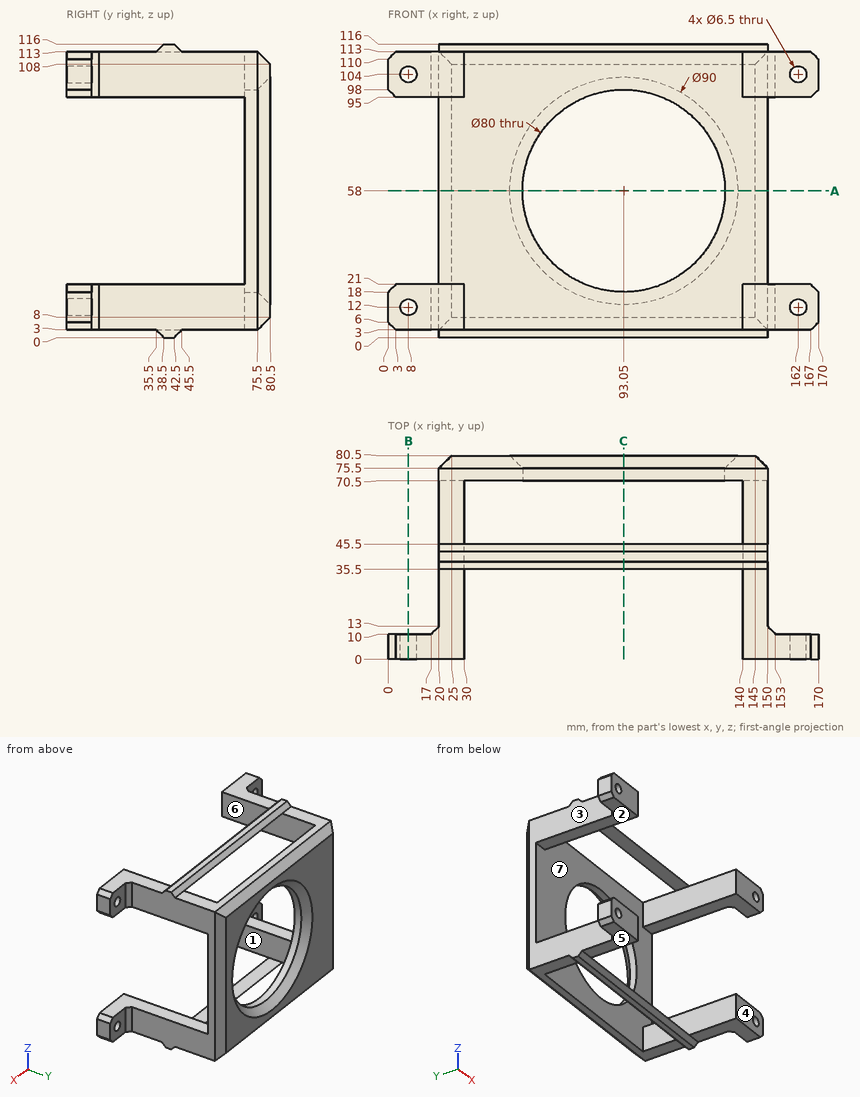
Study the drawing (mm; zero at the part's minimum x, y, z) and answer. A direction names the side the tool comes from. Round coordinates to 2 decimals unless told otherwise and drop trailing zeros. Write each loop counter-clockwise with the first axis right and the second up, starting at its lowest first coordinate (ties: lowest second). Pieces come first, ordered by that corner, then holes. Notation, with made-up numbers: (-34, -23.75) -> (-11, -23.75) arc R17 ccw to (-11, -12.75) -> close; hole circle Ø9 at (41.5, 30). An arc over 180 degrees is marked (long way). Answer as CSV lines item,"result". Start each with the question number.
(1) A tool of negligible diameter and unlimited length cuts with its end or side. For the marked faces 1, 2 and 3, from which of +Z, -Z, +X, -X, +Y, -Y can it reach the whole face along a straight path? Write none if from no direction.
(2) Each of these flat-tipped pins is pushed along its axis until it touches: pin 1 (18.5 mm diameter, centred on x = 9, z = 8.5, fed in from +Y); pin 2 (9 mm diameter, centred on y = 49, z = 101.5, fed in from +X); pin 3 (24 mm diameter, centred on x = 71, y = 67, fed in from +Z). Where does it stop, or does it pass through?
(3) The part is cut by section B-B, the plane x = 8. Give the vertices of the cut face in (y, z).
(4) The part is cut by section C-C, the plane x = 93.05. Give the number of separate pieces and of enclosed holes in the cut face, then the cut area to 3 significant figures.
(5) The part is cut by section A-A, the plane z = 58. Give the vertices of the cut face in (x, y), then the cut area to 3 significant figures.
(6) The mould has two halves that part along Z. Classify the marked faces 4, 5, 6 and 7: +Z half, -Z half, draft (parallel to the pull), parting line (faces both ways), or undercut.
(7) Find the intervals of material crossed by probe 1 along Z at (x, y) = (93.05, 73.5); probe 2 along X at (y, z) = (68.5, 14); probe 3 along Z at (x, y) = (25, 26.5), in increasing order.
Output values:
1,face 1,"-Y"
1,face 2,"+X, -X, -Y"
1,face 3,"+Z, -Z, -X, +Y"
2,pin 1,"stops at y = 11.25"
2,pin 2,"stops at x = 150"
2,pin 3,"stops at z = 113"
3,outline,"(0, 3) -> (10, 3) -> (10, 8.75) -> (0, 8.75) -> close; (0, 15.25) -> (10, 15.25) -> (10, 21) -> (0, 21) -> close; (0, 95) -> (10, 95) -> (10, 100.75) -> (0, 100.75) -> close; (0, 107.25) -> (10, 107.25) -> (10, 113) -> (0, 113) -> close"
4,separate pieces,"4"
4,enclosed holes,"0"
4,area,"292 mm²"
5,outline,"(20, 70.5) -> (53.05, 70.5) -> (53.05, 75.5) -> (48.05, 80.5) -> (25, 80.5) -> (20, 75.5) -> close; (133.05, 70.5) -> (150, 70.5) -> (150, 75.5) -> (145, 80.5) -> (138.05, 80.5) -> (133.05, 75.5) -> close"
5,area,"450 mm²"
6,face 4,"draft"
6,face 5,"-Z half"
6,face 6,"undercut"
6,face 7,"undercut"
7,probe 1,"z = 3 to 18, 98 to 113"
7,probe 2,"x = 20 to 30, 140 to 150"
7,probe 3,"z = 3 to 21, 95 to 113"
